Input: part model. Units: mm. Frame: model coordinates. A direction names the side the tool comes from. Coordinates: 2 decimals unless noted, no trailing zeros. Loops run counter-clockwise (first coordinate to the right, second up) from the corner with the lowest first, then second, coordinate; pieces in that order, holes last.
(1) Set-up query: faces 1 (the face through (-18, -10, 16)), 2 (the face through (-0.57, -15.62, 9.4)), 3 (the face through (-3, -15, 10)). Return all of +Z, -Z, +X, -X, +Y, -Y with unobstructed straight access to the full face (end or side cutting, diameter ignored); none if empty.
(2) Line query: L1, parallel to X at y = -10, z = 7.5; L2, parallel to Y at x = -21, z = 4.75; L3, parallel to Z at x = -12, y = -10.75. Output: solid intervals per line, ascending.
(3) Section C-C, the plane z = 3.5. Return loops of the section in (x, y).
(4) Section B-B, the plane x = -3. Return loops of the section in (y, z), then the cut area to 3 significant figures.
(5) Contact query for flat-ended pins moving along their axis: P1, Ø1.6, axis at x = -21, y = -17.5, coming from the +Z side; P2, Ø12, axis at y = -14, z = 22, coming from the -X side; P3, Ø2.5, axis at y = -6.5, z = 17, coming from the +X side. Output: stop coordinate, or through.
(6) Section A-A, the plane y = -3.25. Return loops of the section in (x, z).
(7) Section D-D, the plane y = -10.5. Give the number of separate pieces and of enclosed holes in the cut face, then the cut area to 3 significant figures.
(8) Mould query, pull axis X, two halves, no side actions, for faces 4 (the face through (-18.6, -15.62, 10.57)), 5 (the face through (-5.4, -15.62, 10.57)), 6 (the face through (-22.5, -10.07, 4.93)), 7 (the face through (-12.14, -18.02, 20.62)). Classes: released by +X, released by -X, zero draft, split by the parting line, or undercut.
```python
from build123d import *

# Parameters (mm, degrees)
PAD_DEPTH      = 20
SKETCH001_R    = 1.5
HOLE_DEPTH     = 25
HOLE_TIPS_R    = 1.5
SKETCH002_R    = 4
HOLE001_DEPTH  = 16
HOLE001_TIPS_R = 4
FILLET_R       = 2


with BuildPart() as part:
    # Sketch → Pad (new body)
    with BuildSketch(Plane.XZ):
        with BuildLine():
            Line((0, 0), (-24, 0))
            Line((-24, 0), (-24, 10))
            Line((-24, 10), (-18, 10))
            Line((-18, 10), (-18, 20))
            ThreePointArc((-6, 20), (-12, 26), (-18, 20))
            Line((-6, 20), (-6, 10))
            Line((-6, 10), (0, 10))
            Line((0, 10), (0, 0))
        make_face()
    extrude(amount=PAD_DEPTH)

    # Sketch001 (on Face4 of Pad) → Hole (cut)
    with BuildSketch(Plane(origin=(0, 0, 0), x_dir=(1, 0, 0), z_dir=(0, 0, -1))):
        with Locations((-21, 10)):
            Circle(SKETCH001_R)
        with Locations((-3, 10)):
            Circle(SKETCH001_R)
    extrude(amount=-HOLE_DEPTH, mode=Mode.SUBTRACT)

    # Hole tips → Hole tip 1 section 0
    with BuildSketch(Plane(origin=(0, 0, 25), x_dir=(1, 0, 0), z_dir=(0, 0, -1)), mode=Mode.PRIVATE) as hole_tip_1_s0:
        with Locations((-21, 10)):
            Circle(HOLE_TIPS_R)
    loft([hole_tip_1_s0.sketch, Vertex(-21, -10, 25.901291)], mode=Mode.SUBTRACT)

    # Hole tips → Hole tip 2 section 0
    with BuildSketch(Plane(origin=(0, 0, 25), x_dir=(1, 0, 0), z_dir=(0, 0, -1)), mode=Mode.PRIVATE) as hole_tip_2_s0:
        with Locations((-3, 10)):
            Circle(HOLE_TIPS_R)
    loft([hole_tip_2_s0.sketch, Vertex(-3, -10, 25.901291)], mode=Mode.SUBTRACT)

    # Sketch002 (on Face4 of Hole) → Hole001 (cut)
    with BuildSketch(Plane(origin=(0, 0, 0), x_dir=(1, 0, 0), z_dir=(0, 1, 0))):
        with Locations((-12, -20)):
            Circle(SKETCH002_R)
    extrude(amount=-HOLE001_DEPTH, mode=Mode.SUBTRACT)

    # Hole001 tips → Hole001 tip 1 section 0
    with BuildSketch(Plane(origin=(0, -16, 0), x_dir=(1, 0, 0), z_dir=(0, 1, 0)), mode=Mode.PRIVATE) as hole001_tip_1_s0:
        with Locations((-12, -20)):
            Circle(HOLE001_TIPS_R)
    loft([hole001_tip_1_s0.sketch, Vertex(-12, -18.403442, 20)], mode=Mode.SUBTRACT)

    # Fillet
    fillet_edges = [part.edges().sort_by_distance(p)[0] for p in [
        (0, -10, 10),
        (-6, -10, 10),
        (-24, -10, 10),
        (-18, -10, 10),
    ]]
    fillet(fillet_edges, radius=FILLET_R)


solid = part.part
```
Report:
1. face 1: +Z, -X, +Y, -Y
1. face 2: +Z, +X, -Y
1. face 3: +Z, +X, +Y, -Y
2. L1: x = -24 to -22.5, -19.5 to -4.5, -1.5 to 0
2. L2: y = -20 to -11.5, -8.5 to 0
2. L3: z = 0 to 16, 24 to 26
3. outline: (-24, -20) - (0, -20) - (0, 0) - (-24, 0) - close; hole circle Ø3 at (-21, -10); hole circle Ø3 at (-3, -10)
4. outline: (-20, 0) - (-11.5, 0) - (-11.5, 10) - (-20, 10) - close; (-8.5, 0) - (0, 0) - (0, 10) - (-8.5, 10) - close
4. area: 170 mm2
5. P1: stops at z = 10
5. P2: stops at x = -18
5. P3: stops at x = -6
6. outline: (-24, 0) - (0, 0) - (0, 8) arc R2 ccw to (-2, 10) - (-4, 10) arc R2 cw to (-6, 12) - (-6, 20) arc R6 ccw to (-18, 20) - (-18, 12) arc R2 cw to (-20, 10) - (-22, 10) arc R2 ccw to (-24, 8) - close; hole circle Ø8 at (-12, 20)
7. separate pieces: 3
7. enclosed holes: 1
7. area: 310 mm2
8. face 4: released by -X
8. face 5: released by +X
8. face 6: undercut
8. face 7: undercut
